from build123d import *

# Parameters (mm, degrees)
F1_DEPTH      = 114
F3_DEPTH      = 10
F4_ANGLE      = 35
F9_T4_DEPTH   = 262.5652555071
F9_S5_R       = 167.9439583926
F9_T6_DEPTH   = 133
F9_S7_R       = 167.9439583926
F9_T8_DEPTH   = 133
F10_T4_DEPTH  = 262.4928960507
F10_S7_R      = 167.9439583926
F10_T8_DEPTH  = 133
F10_S9_R      = 167.9439583926
F10_T10_DEPTH = 133


# Not quite as in the source:
# - a fillet or chamfer that OpenCascade refuses, or shapes differently, is made with other operations: its cross-section is extruded or revolved along the edge and cut away or added


with BuildPart() as f1:
    # F0 (on Front) → F1 (new body, symmetric)
    with BuildSketch(Plane.XZ):
        with BuildLine():
            ThreePointArc((-332.1381211281, 0), (12.8618788719, 35.0482151539), (357.8618788719, 0))
            Line((357.8618788719, 0), (357.8618788719, 10))
            ThreePointArc((357.8618788719, 10), (12.8618788719, 45.0482151539), (-332.1381211281, 10))
            Line((-332.1381211281, 10), (-332.1381211281, 0))
        make_face()
    extrude(amount=F1_DEPTH, both=True)


with BuildPart() as f3:
    # F2 (on Top) → F3 (new body)
    with BuildSketch(Plane.XY):
        with BuildLine():
            ThreePointArc((123.1073781215, 58.2170858979), (58.6810369853, 73.3595252621), (5.1073781215, 112.2170853764))
            Line((5.1073781215, 112.2170853764), (5.1073781215, -115.7829146236))
            ThreePointArc((5.1073781215, -115.7829146236), (58.6810369853, -76.9253545093), (123.1073781215, -61.7829151452))
            Line((123.1073781215, -61.7829151452), (123.1073781215, 58.2170858979))
        make_face()
    extrude(amount=F3_DEPTH)


with BuildPart() as f3_1:
    # F4: moved
    add(f3.part.rotate(Axis((5.1073781215, -1.7829146236, 0), (0, -1, 0)), F4_ANGLE))


with BuildPart() as f3_2:
    # F5: moved
    add(f3_1.part.moved(Location((352.9, 1.9, 0))))


with BuildPart() as f6_1:
    # F6: instance of F3
    add(f3_2.part.mirror(Plane.YZ))


with BuildPart() as f6_1_1:
    # F7: moved
    add(f6_1.part.moved(Location((25.6, 0, 0))))

    # F8: union F1, F3
    add(f1.part)
    add(f3_2.part)

    # F9: fillet of radius 20 on 1 edges, made by hand


with BuildPart() as f9_tool2:
    # F9_s3 → F9_t4 (new body)
    with BuildSketch(Plane.XZ.offset(-131.39971313)):
        with BuildLine():
            add(Edge.make_bspline(
                [(-336.9253398984, 15.3712567812), (-329.9304765428, 10.4734007308), (-321.5551366342, 12.1379693445)],
                knots=[0, 0, 0, 1, 1, 1], degree=2, weights=[1, 1, 1]))
            ThreePointArc((-321.5551366342, 12.1379693445), (-325.7318557218, 11.3024702142), (-329.9064875028, 10.4566034242))
            Line((-329.9064875028, 10.4566034242), (-336.9253398984, 15.3712567812))
        make_face()
    extrude(amount=F9_T4_DEPTH)

    # F9_s5 → F9_t6 (cut, symmetric)
    with BuildSketch(Plane(origin=(-102.2686786014, 0, -146.0548094967), x_dir=(0, 1, 0), z_dir=(-0.5735764364, 0, -0.8191520443))):
        with Locations((-227.7381227134, -395.7513456072)):
            Circle(F9_S5_R)
    extrude(amount=F9_T6_DEPTH, both=True, mode=Mode.SUBTRACT)

    # F9_s7 → F9_t8 (cut, symmetric)
    with BuildSketch(Plane(origin=(-102.2686786014, 0, -146.0548094967), x_dir=(0, 1, 0), z_dir=(-0.5735764364, 0, -0.8191520443))):
        with Locations((227.9722934661, -395.7513456072)):
            Circle(F9_S7_R)
    extrude(amount=F9_T8_DEPTH, both=True, mode=Mode.SUBTRACT)

    split(bisect_by=Plane.XZ.offset(114), keep=Keep.BOTTOM)

    split(bisect_by=Plane.XZ.offset(-114), keep=Keep.TOP)


with BuildPart() as f6_1_2:
    add(f6_1_1.part)

    # F9_t1: union F9_tool2
    add(f9_tool2.part)

    # F10: fillet of radius 20 on 1 edges, made by hand


with BuildPart() as f10_tool2:
    # F10_s3 → F10_t4 (new body)
    with BuildSketch(Plane.XZ.offset(-131.3635334017)):
        with BuildLine():
            add(Edge.make_bspline(
                [(347.1836055083, 12.1569048592), (355.5583829749, 10.492941025), (362.5526978832, 15.3904130484)],
                knots=[0, 0, 0, 1, 1, 1], degree=2, weights=[1, 1, 1]))
            Line((362.5526978832, 15.3904130484), (355.5343963998, 10.4761454443))
            ThreePointArc((355.5343963998, 10.4761454443), (351.360044149, 11.3217082271), (347.1836055083, 12.1569048592))
        make_face()
    extrude(amount=F10_T4_DEPTH)

    split(bisect_by=Plane.XZ.offset(114), keep=Keep.BOTTOM)

    split(bisect_by=Plane.XZ.offset(-114), keep=Keep.TOP)

    # F10_s7 → F10_t8 (cut, symmetric)
    with BuildSketch(Plane(origin=(110.6428945721, 0, -158.0144293433), x_dir=(0, 1, 0), z_dir=(0.5735764364, 0, -0.8191520443))):
        with Locations((227.9722934661, 416.721637941)):
            Circle(F10_S7_R)
    extrude(amount=F10_T8_DEPTH, both=True, mode=Mode.SUBTRACT)

    # F10_s9 → F10_t10 (cut, symmetric)
    with BuildSketch(Plane(origin=(110.6428945721, 0, -158.0144293433), x_dir=(0, 1, 0), z_dir=(0.5735764364, 0, -0.8191520443))):
        with Locations((-227.7381227134, 416.721637941)):
            Circle(F10_S9_R)
    extrude(amount=F10_T10_DEPTH, both=True, mode=Mode.SUBTRACT)


with BuildPart() as f6_1_3:
    add(f6_1_2.part)

    # F10_t1: union F10_tool2
    add(f10_tool2.part)


solid = f6_1_3.part
Verification items for the finished model (mm, model axes). A direction names the side the tool comes from. Give positions to 0.01 mm unless a question says otherwise; leave off trailing zeros. Write each loop counter-clockwise with the first axis right and the second up, starting at its lowest first coordinate (ties: lowest second). Pieces come first, ordered by that corner, then holes.
(1) Access from +Z, -Z, +X, -X, +Y, -Y to the whole of each face (thin tool, end or side, straight path). Record for faces 1 (the face through (-369.321, 1.713, 25.847)), 2 (the face through (405.14, 1.54, 45.21)).
(2) Gauge pin test, flat ends, axial feed: pin 1 (10 mm diameter, centred on x = 330, y = -35.5, fed in from -Z); pin 2 (4.5 mm diameter, centred on y = 110, z = 5, fed in from +X); pin 3 (1.5 mm diameter, centred on y = 55.5, z = 41, fed in from +X). Record the tip position at first contact, or that the pin passes through.
(3) Cross-section at A-A (x = 312). Enter the section's corners in (y, z).
(4) Material ranges on line 1 (X direction, y = -47, z = 69); line 2 (Z direction, x = -3.5, y = -22); line 3 (Z direction, x = -274, y = -70), recorded low to high.
(5) Mould release check, pull along X, two halves, no side actions. Record for faces 3 (the face through (-379.524, 1.542, 45.199)), 4 (the face through (11, -114, 38)), 5 (the face through (394.921, 1.713, 25.847)): +X half, -X half, draft (parallel to the pull), parting line (faces both ways), or undercut.
Worked out:
1. face 1: -Z, -X, +Y, -Y
1. face 2: +Z, +Y, -Y
2. pin 1: stops at z = 4.53
2. pin 2: stops at x = 362.48
2. pin 3: stops at x = 417.63
3. outline: (-114, 8.77) - (114, 8.77) - (114, 18.77) - (-114, 18.77) - close
4. line 1: x = -428.14 to -413.52, 439.12 to 453.74
4. line 2: z = 34.97 to 44.97
4. line 3: z = 10.89 to 20.89
5. face 3: undercut
5. face 4: draft
5. face 5: +X half
